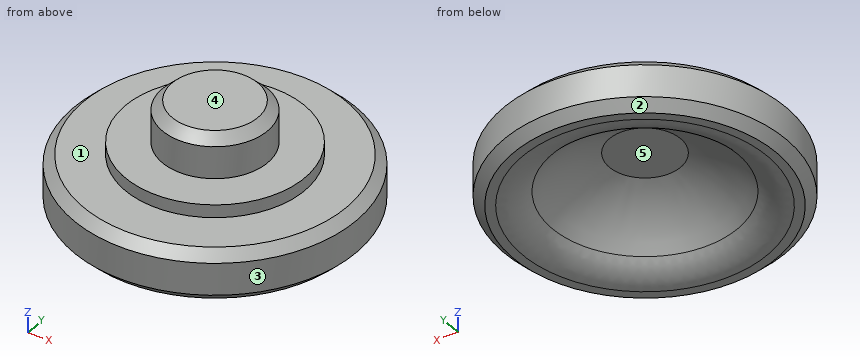
```python
from build123d import *

# Parameters (mm, degrees)
F2_R    = 3
F3_SIZE = 0.75
F4_SIZE = 0.75


with BuildPart() as f1:
    # F0 (on Front) → F1 (revolve)
    with BuildSketch(Plane.XZ):
        with BuildLine():
            Line((-11, -1.722947), (-11, -5.722947))
            Line((-11, -5.722947), (-8, -5.722947))
            ThreePointArc((-8, -5.722947), (-5.767763, -3.181992), (-2.775571, -1.605249))
            Line((-2.775571, -1.605249), (0, -1.605249))
            Line((0, -1.605249), (0, 2.527053))
            Line((0, 2.527053), (-4.1, 2.527053))
            Line((-4.1, 2.527053), (-4.1, -0.722947))
            Line((-4.1, -0.722947), (-7, -0.722947))
            Line((-7, -0.722947), (-7, -1.722947))
            Line((-7, -1.722947), (-11, -1.722947))
        make_face()
    revolve(axis=Axis((0, 0, -0.8276), (0, 0, -1)))

    # F2
    f2_edges = [f1.edges().sort_by_distance(p)[0] for p in [
        (8, 0, -5.722947),
    ]]
    fillet(f2_edges, radius=F2_R)

    # F3
    f3_edges = [f1.edges().sort_by_distance(p)[0] for p in [
        (11, 0, -5.722947),
        (11, 0, -1.722947),
    ]]
    chamfer(f3_edges, length=F3_SIZE)

    # F4
    f4_edges = [f1.edges().sort_by_distance(p)[0] for p in [
        (4.1, 0, 2.527053),
    ]]
    chamfer(f4_edges, length=F4_SIZE)


solid = f1.part
```
Input: part model. Units: mm. Frame: model coordinates. Face numbers are marked on the shaded views. A direction names the side the tool comes from. Round coordinates to 2 decimals unless told otherwise and drop trailing zeros. Write each loop counter-clockwise with the first axis right and the second up, starting at its lowest first coordinate (ties: lowest second). Pieces come first, ordered by that corner, then holes. Notation, with made-up numbers: M 16.5,43 L 58.5,43 A7 cw 58.5,48 Z; hole C 79,-15.75 d4. An arc over 180 degrees is marked long. Write each question's results on one line, items separated by ' | '.
Q1. Access query for the marked faces 1 and 2. Directions: +Z, -Z, +X, -X, +Y, -Y. A direction counts if a zero-diameter tool reaches every point of the face in a straight line with its end or side. Return the directions, or none.
Results:
face 1: +Z | face 2: -Z
Q2. Line query: line 1 along Y through (x, z) = (6, -4.5); line 2 along Y through (x, z) = (0.5, -3.75); line 3 along Y through (x, z) = (8, -4.25). Output: solid intervals per line, ascending.
Results:
line 1: y = -9.22 to -3.85, 3.85 to 9.22 | line 2: y = -10.99 to -6.4, 6.4 to 10.99 | line 3: y = -7.55 to 7.55
Q3. Pin query (flat end, axial travel): P1, Ø1.5, axis at x = 0, y = 8, coming from the -Z side; P2, Ø1, axis at y = -3, z = -1, coming from the -X side; P3, Ø1.7, axis at x = 0.5, y = 0.5, coming from the -Z side. Return the tip coordinate at first contact, or that it passes through.
Results:
P1: stops at z = -5.61 | P2: stops at x = -6.54 | P3: stops at z = -1.61
Q4. Section query A-A (z = 1.5). Return loops of the section in (x, y).
Results:
outline: C 0,0 d8.2
Q5. Draft query along Y for the marked faces 3, 4 and 5. Return one class per face: released by +Y, released by -Y, zero draft, split by the parting line, or undercut.
Results:
face 3: split by the parting line | face 4: zero draft | face 5: undercut
